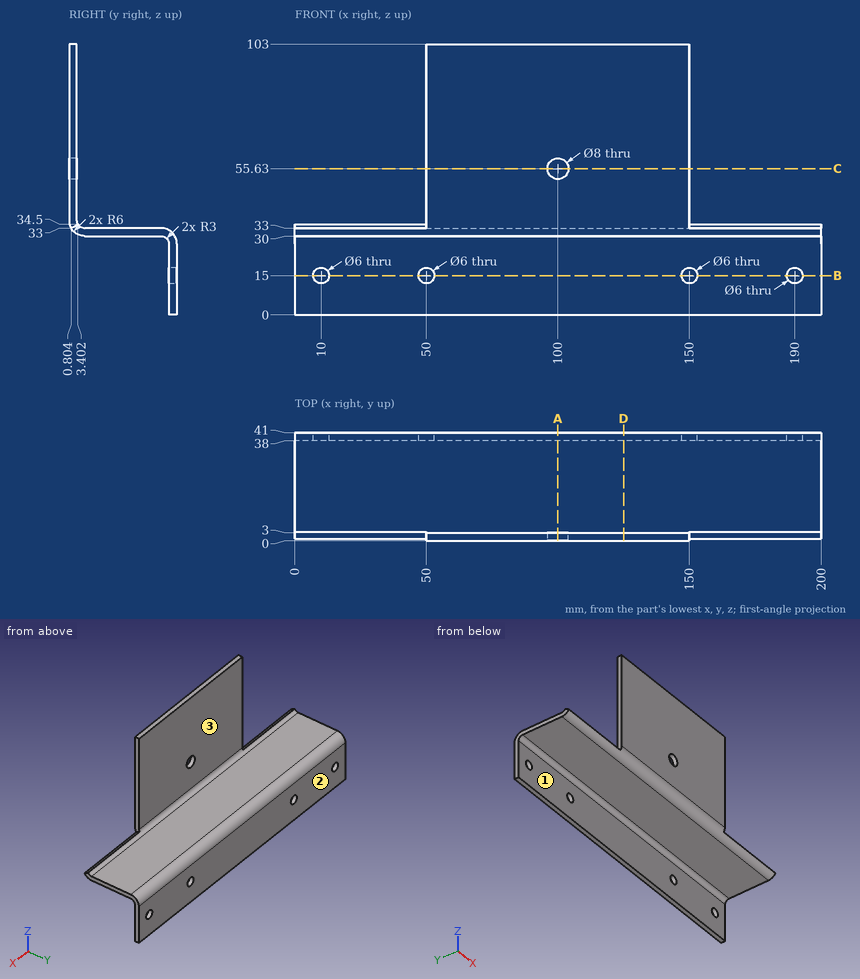
Answer from the drawing. Dimensions are ordinates in mm from the lowest x, y and z of the part. A direction names the side the tool comes from. Coordinates: 2 decimals unless noted, no trailing zeros. Order: outer loops, then holes, each group sorted by start corner. A loop starts at its lowest first (then second) coordinate and runs counter-clockwise, first axis right, second up. Notation, with made-up numbers: (67.25, 2) - (99.25, 2) arc R12 ccw to (99.25, 16) - close; hole circle Ø3 at (89, 53). An arc over 180 degrees is marked (long way). Use one line per item in the form item = value.
(1) Straight lines are drawn through the part: L1, parallel to X at y = 40, z = 15; L2, parallel to Y at x = 93.5, z = 40; L3, parallel to Z at x = 176, y = 19.5. For each, find the intervals that lie inside material, in ascending order.
Computed values:
L1 = 0 to 7, 13 to 47, 53 to 147, 153 to 187, 193 to 200
L2 = 0 to 3
L3 = 30 to 33
(2) Section A-A, the plane x = 100 is taken. Give the vertices of the cut face in (y, z), then the cut area to 3 significant figures.
Computed values:
outline = (0, 36) arc R6 ccw to (6, 30) - (35, 30) arc R3 cw to (38, 27) - (38, 0) - (41, 0) - (41, 27) arc R6 ccw to (35, 33) - (6, 33) arc R3 cw to (3, 36) - (3, 51.63) - (0, 51.63) - close; (0, 59.63) - (3, 59.63) - (3, 103) - (0, 103) - close
area = 387 mm²
(3) Given pin 1 Ø5 at (x, z) = (150, 15) entering from -Y (3 decimals); pin 2 Ø7 at (x, z) = (10, 15) entering from +Y; pin 3 Ø1 at (x, z) = (140, 87) entering from +Y; pin 4 Ø23 at (x, y) = (51, 23) entering from +Z, each flat-ended and moving along its own axis, determine where each tip first touches the part or whether it passes through.
Computed values:
pin_1 = through
pin_2 = 41
pin_3 = 3
pin_4 = 33
(4) Section D-D, the plane x = 125 is taken. Give the vertices of the cut face in (y, z).
Computed values:
outline = (0, 36) arc R6 ccw to (6, 30) - (35, 30) arc R3 cw to (38, 27) - (38, 0) - (41, 0) - (41, 27) arc R6 ccw to (35, 33) - (6, 33) arc R3 cw to (3, 36) - (3, 103) - (0, 103) - close
(5) Section B-B, the plane z = 15 is taken. Give the vertices of the cut face in (x, y), then the cut area to 3 significant figures.
Computed values:
outline = (0, 38) - (7, 38) - (7, 41) - (0, 41) - close; (13, 38) - (47, 38) - (47, 41) - (13, 41) - close; (53, 38) - (147, 38) - (147, 41) - (53, 41) - close; (153, 38) - (187, 38) - (187, 41) - (153, 41) - close; (193, 38) - (200, 38) - (200, 41) - (193, 41) - close
area = 528 mm²
(6) Which of the six approach directions +Z, -Z, +X, -X, +Y, -Y give full straight-line access (tool end or side, diameter ignored) to the marked faces 1, 2 and 3?
Computed values:
face_1 = -Z, +X, -X, -Y
face_2 = +Z, -Z, +X, -X, +Y
face_3 = +Z, +X, -X, +Y
(7) Section C-C, the plane z = 55.63 is taken. Give the vertices of the cut face in (x, y), then the cut area to 3 significant figures.
Computed values:
outline = (50, 0) - (96, 0) - (96, 3) - (50, 3) - close; (104, 0) - (150, 0) - (150, 3) - (104, 3) - close
area = 276 mm²
